Here's how the part is built. I have some questions about the finished solid (model axes, mm). Coordinates: 2 decimals unless noted, no trailing zeros. Write each loop counter-clockwise with the first axis right and the second up, starting at its lowest first coordinate (ties: lowest second). Pieces come first, ordered by that corner, then holes. Notation, with made-up numbers: (44.5, 28.5) -> (93.5, 28.5) arc R21 cw to (93.5, 44.5) -> close; hole circle Ø11 at (12, -1). An arc over 180 degrees is marked (long way). Use a Markdown table: item, result. Add a question column.
Item 1: Imagine slicing it at B-B, the plane x = -9.25. Write out the boundary of the cut face in (y, z).
Item 2: Imagine slicing it at A-A, the plane z = -27. Write out the boundary of the cut face in (x, y).
Item 3: If I drill on line 1 along Z through (x, y) = (9.25, 3.25); line 2 along Z through (x, y) = (-8.25, -4), over which ranges is the centre line in solid material (lowest first)? Write a range as from..to.
Item 4: Will this pin go through, and if not, where does the flat tip stop? pin 1 Ø1.5 at (x, z) = (-9.25, 29) entering from -Y.
Item 5: If we mould it in two halves opening along Z, with no side actions, what happens to faces 1 (the cylindrical face through (10.5, 0.15, -26.95)), 2 (the flat face through (0, 0, -32)), 3 (the flat face through (13, 0, 0))? For each: pulls with the +Z half, pulls with the -Z half, needs draft (parallel to the pull), parting line crosses it, or undercut.
```python
from build123d import *

# Parameters (mm, degrees)
SKETCH_1_W          = 26
SKETCH_1_H          = 22
EXTRUDE_1_DEPTH     = 32
SKETCH_2_R          = 1.25
CUT_EXTRUDE_1_DEPTH = 40


with BuildPart() as part:
    # 草图1 → 凸台-拉伸1 (new, symmetric)
    with BuildSketch(Plane.XY):
        Rectangle(SKETCH_1_W, SKETCH_1_H)
    extrude(amount=EXTRUDE_1_DEPTH, both=True)

    # 草图2 → 切除-拉伸1 (cut)
    with BuildSketch(Plane(origin=(0, 11, 0), x_dir=(1, 0, 0), z_dir=(0, 1, 0))):
        with Locations(Location((9.25, -29, 0), (0, 0, 180))):
            Circle(SKETCH_2_R)
        with Locations(Location((9.25, 27, 0), (0, 0, 180))):
            Circle(SKETCH_2_R)
        with Locations(Location((-9.25, 27, 0), (0, 0, 180))):
            Circle(SKETCH_2_R)
        with Locations(Location((-9.25, -29, 0), (0, 0, 180))):
            Circle(SKETCH_2_R)
    extrude(amount=-CUT_EXTRUDE_1_DEPTH, mode=Mode.SUBTRACT)


solid = part.part
```
Ans:
| question | item | result |
|---|---|---|
| 1 | outline | (-11, -32) -> (11, -32) -> (11, -28.25) -> (-11, -28.25) -> close; (-11, -25.75) -> (11, -25.75) -> (11, 27.75) -> (-11, 27.75) -> close; (-11, 30.25) -> (11, 30.25) -> (11, 32) -> (-11, 32) -> close |
| 2 | outline | (-13, -11) -> (-10.5, -11) -> (-10.5, 11) -> (-13, 11) -> close; (-8, -11) -> (8, -11) -> (8, 11) -> (-8, 11) -> close; (10.5, -11) -> (13, -11) -> (13, 11) -> (10.5, 11) -> close |
| 3 | line 1 | z = -32..-28.25, -25.75..27.75, 30.25..32 |
| 3 | line 2 | z = -32..-27.75, -26.25..28.25, 29.75..32 |
| 4 | pin 1 | passes through |
| 5 | face 1 | undercut |
| 5 | face 2 | pulls with the -Z half |
| 5 | face 3 | needs draft |
